Build history of the part. All positions in model axes, mm. A direction names the side the tool comes from. Round coordinates to 2 decimals unless told otherwise and drop trailing zeros. Order: outer loops, then holes, each group sorted by start corner. A loop starts at its lowest first (then second) coordinate and runs counter-clockwise, first axis right, second up. Notation, with made-up numbers: (8.5, 17) -> (19.5, 17) arc R20 cw to (19.5, 43) -> close; hole circle Ø3 at (88, -29). An arc over 180 degrees is marked (long way). Use a Markdown table: item, result. Add a question column.
Item 1: Slice it at B-B, the plane y = 30. Give the cut face in (x, z).
Item 2: Two-plate mould, pull along Y, no slides. Class faces 1 (the face through (14.01, 46.8, 2.03)), 2 (the face through (24.615, 12.917, 1.972)), 3 (the face through (28.755, 45.919, 2.028)): released by +Y, released by -Y, zero draft, split by the parting line, or undercut.
Item 3: Slice it at A-A, the plane x = 0. Give the cut face in (y, z), plus the area to 3 significant figures.
Item 4: Pin check, flat tip, straight feed: pin 1 (2 mm diameter, centred on x = 10, y = 19, fed in from -Z). Stop position of the tip, or through.
Item 5: Probe L1, parallel to X at y = 5, z = 2.1; L2, parallel to X at y = 35, z = 0.6; L3, parallel to Y at x = 23, z = 1. List the from-to ranges inside material, lowest first.
Item 6: 3-axis set-ups, long thin cutter, end or side, ignore diameter. For faces 4 (the face through (9.742, 20.967, 1.972)), 5 (the face through (26.25, 58.82, 1.97)): which of +Z, -Z, +X, -X, +Y, -Y reach the whole face in a straight line?
Autodesk Inventor part; units mm, degrees
ref_plane "YZ Plane" through (0, 0, 0) normal (1, 0, 0) x (0, 1, 0)
ref_plane "XZ Plane" through (0, 0, 0) normal (0, 1, 0) x (-1, 0, 0)
ref_plane "XY Plane" through (0, 0, 0) normal (0, 0, 1) x (1, 0, 0)
sketch "Body" plane through (0, 0, 0) normal (0, 0, 1) x (1, 0, 0)
  line L0 (28.8487, 38.4543) -> (2.7256, -1.7701)
  line L1 (22.3487, 40.3798) -> (-2.7256, 1.7701)
  line L2 (22.3487, 40.3798) -> (22.3487, 45.0293)
  line L3 (28.8487, 38.4543) -> (28.8487, 45.9543)
  line L4 (32.4946, 58.4071) -> (39.19, 35.3599)
  line L5 (19.5232, 59.2689) -> (32.4946, 58.4071)
  line L6 (14.1445, 46.7648) -> (14.7577, 52.2305)
  line L7 (22.3487, 45.0293) -> (20.7935, 50.3829) construction
  line L8 (28.8487, 45.9543) -> (27.0354, 52.1963) construction
  arc A0 (-11.4127, 7.4118) -> (11.4127, -7.4118) centre (0, 0) ccw
  line L9 (-11.4127, 7.4118) -> (14.1445, 46.7648)
  line L10 (11.4127, -7.4118) -> (39.19, 35.3599)
  circle A1 centre (0, 0) radius 3.25
  line L11 (25.5987, 39.4171) -> (0, 0) construction
  line L12 (25.5987, 39.4171) -> (25.5987, 45.4918) construction
  line L13 (25.5987, 45.4918) -> (24.7618, 48.3727) construction
  line L14 (19.5232, 59.2689) -> (14.7577, 52.2305)
  line L15 (-30.4273, 0) -> (50.7929, 0) construction
  line L16 (20.7935, 50.3829) -> (22.2339, 50.8014) construction
  line L17 (22.3487, 45.0293) -> (22.2339, 50.8014)
  line L18 (28.8487, 45.9543) -> (25.595, 51.7778)
  line L19 (22.2339, 50.8014) -> (25.595, 51.7778)
  line L20 (25.595, 51.7778) -> (27.0354, 52.1963) construction
  dimension "d37" = 6.5
  dimension "d38" = 130.8
  dimension "d45" = 3.25
  dimension "d46" = 3.25
  dimension "d47" = 3.25
  dimension "d48" = 3.25
  dimension "d49" = 3.25
  dimension "d50" = 3.25
  dimension "d51" = 47
  dimension "d52" = 7.5
  dimension "d54" = 123.001
  dimension "d56" = 130.8
  dimension "d57" = 24
  dimension "d58" = 13
  dimension "d59" = 8.5
  dimension "d60" = 5.5
  dimension "d61" = 110
  dimension "d62" = 120.3
  dimension "d63" = 51
  dimension "d64" = 153.4
  dimension "d74" = 6.5
  dimension "d75" = 1.5
  dimension "d76" = 1.5
extrude "BodyFeature" add sketch "Body" along normal blind 4
fillet "BodyFillet1Feature" radius 3.5 1 edges at (19.5232, 59.2689, 2)
fillet "BodyFillet2Feature" radius 5 1 edges at (14.7577, 52.2305, 2)
fillet "BodyFillet3Feature" radius 2 1 edges at (32.4946, 58.4071, 2)
fillet "BodyFillet4Feature" radius 4 1 edges at (39.19, 35.3599, 2)
fillet "BodyFillet5Feature" radius 5 1 edges at (14.1445, 46.7648, 2)
fillet "InsideFilletsFeature" radius 3 4 edges at (22.3487, 40.3798, 2) (22.3487, 45.0293, 2) (28.8487, 45.9543, 2) (28.8487, 38.4543, 2)
fillet "InsideFilletsSmallFeature" radius 1 2 edges at (22.2339, 50.8014, 2) (25.595, 51.7778, 2)
properties part number "PelvisLinkLeft"
Check sheet entries:
| question | item | result |
|---|---|---|
| 1 | outline | (3.26, 0) -> (15.61, 0) -> (15.61, 4) -> (3.26, 4) -> close; (23.36, 0) -> (35.71, 0) -> (35.71, 4) -> (23.36, 4) -> close |
| 2 | face 1 | released by +Y |
| 2 | face 2 | released by -Y |
| 2 | face 3 | undercut |
| 3 | outline | (-13.61, 0) -> (-3.25, 0) -> (-3.25, 4) -> (-13.61, 4) -> close; (5.97, 0) -> (24.99, 0) -> (24.99, 4) -> (5.97, 4) -> close |
| 3 | area | 118 mm2 |
| 4 | pin 1 | through |
| 5 | L1 | -12.66 to -0.63, 7.12 to 19.47 |
| 5 | L2 | 6.5 to 18.85, 26.61 to 38.71 |
| 5 | L3 | 10.43 to 29.45, 51.02 to 59.04 |
| 6 | face 4 | +Z, -Z |
| 6 | face 5 | +Z, -Z, +X, +Y |
